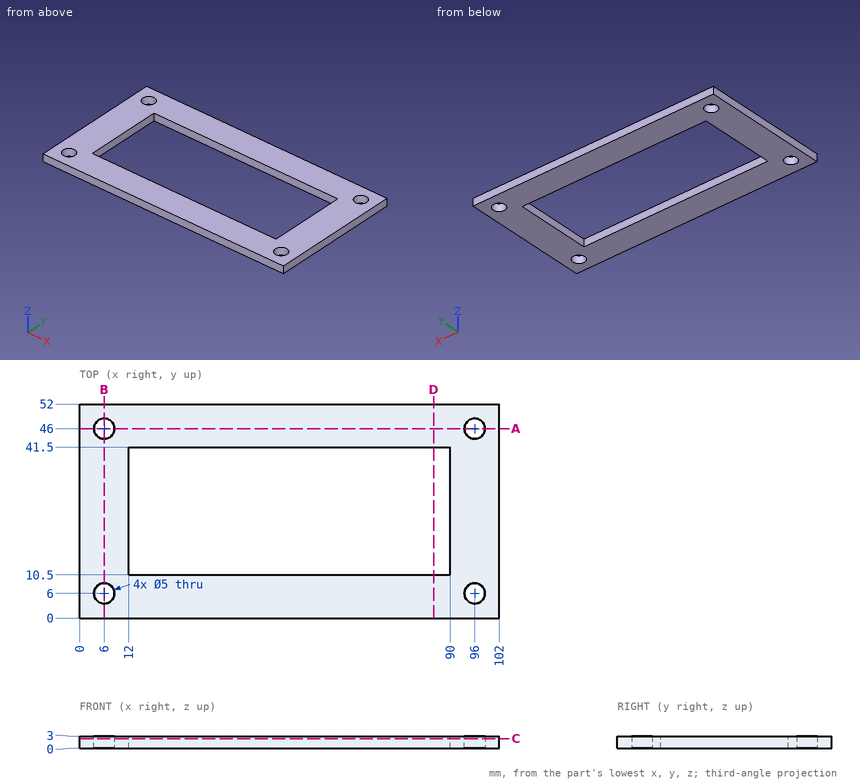
Can you work these out from the drawing? Everything is in mm from the part's minimum corner. Coordinates: 2 decimals unless noted, no trailing zeros. Order: outer loops, then holes, each group sorted by start corner. A loop starts at its lowest first (then second) coordinate and runs counter-clockwise, first axis right, second up. Notation, with made-up numbers: M 72.5,33 L 92.5,33 A15 cw 92.5,60 Z; hole C 64.25,-3 d10. An arc over 180 degrees is marked long. Answer as CSV lines item,"result". Start each with the question number.
1. I want a section at C-C, the plane z = 2.4. Write out the boundary of the cut face in (x, y).
2. I want a section at D-D, the plane x = 86. Write out the boundary of the cut face in (y, z), and give its area (3 significant figures).
3. I need wall thicknesses on line 1 (Y direction, x = 6, z = 2.3); line 2 (X direction, y = 46, z = 2); line 3 (Y direction, x = 56, z = 0.25). Which ranges of each line are inside material? Lowest first, please. Write a range as [from, to].
4. I want a section at A-A, the plane y = 46. Write out the boundary of the cut face in (x, z), and give its area (3 significant figures).
5. I want a section at B-B, the plane x = 6. Write out the boundary of the cut face in (y, z), and give its area (3 significant figures).
Recorded:
1,outline,"M 0,0 L 102,0 L 102,52 L 0,52 Z; hole C 6,6 d5; hole C 6,46 d5; hole M 12,10.5 L 90,10.5 L 90,41.5 L 12,41.5 Z; hole C 96,6 d5; hole C 96,46 d5"
2,outline,"M 0,0 L 10.5,0 L 10.5,3 L 0,3 Z; M 41.5,0 L 52,0 L 52,3 L 41.5,3 Z"
2,area,"63.0 mm2"
3,line 1,"y = [0, 3.5], [8.5, 43.5], [48.5, 52]"
3,line 2,"x = [0, 3.5], [8.5, 93.5], [98.5, 102]"
3,line 3,"y = [0, 10.5], [41.5, 52]"
4,outline,"M 0,0 L 3.5,0 L 3.5,3 L 0,3 Z; M 8.5,0 L 93.5,0 L 93.5,3 L 8.5,3 Z; M 98.5,0 L 102,0 L 102,3 L 98.5,3 Z"
4,area,"276 mm2"
5,outline,"M 0,0 L 3.5,0 L 3.5,3 L 0,3 Z; M 8.5,0 L 43.5,0 L 43.5,3 L 8.5,3 Z; M 48.5,0 L 52,0 L 52,3 L 48.5,3 Z"
5,area,"126 mm2"
